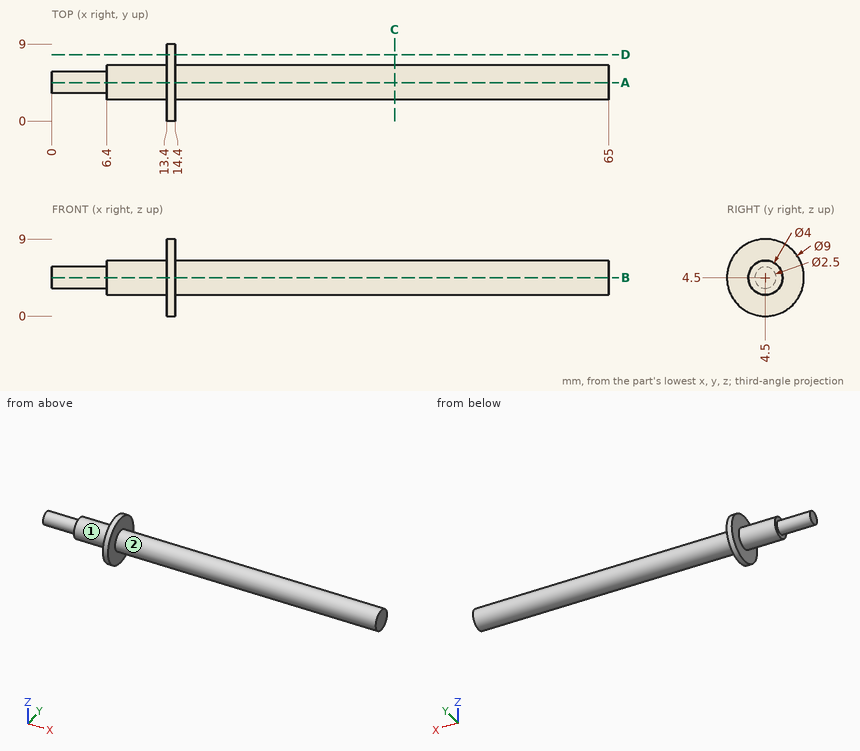
Geometry check sheet. Reference: drawing and pictorial views, mm from the part's lowest x, y, z. A direction names the side the tool comes from. Coordinates: 2 decimals unless noted, no trailing zeros. Write each loop counter-clockwise with the first axis right and the second up, starting at its lowest first coordinate (ties: lowest second). Pieces come first, ordered by that corner, then holes. Notation, with made-up numbers: (-2, 35.5) - (2, 35.5) arc R16 ccw to (2, 50.5) - close; hole circle Ø11 at (64, 48.5). An arc over 180 degrees is marked (long way). One line per question, with ' | ' between items. Start each with the question number.
1. Section check A-A (y = 4.5). Enter the section's corners in (x, z).
2. Material ranges on line 1 along X through (y, z) = (3, 6.5); line 2 along X through (y, z) = (5.75, 3.25); line 3 along Y through (x, z) = (49.5, 3.75), recorded low to high.
3. Gauge pin test, flat ends, axial feed: P1, Ø1.5, axis at y = 3.5, z = 5, coming from the -X side; P2, Ø1.5, axis at x = 20, y = 5.5, coming from the +Z side; P3, Ø1.5, axis at y = 6, z = 1.5, coming from the +X side; P4, Ø2, axis at x = 7.5, y = 4, coming from the -Z side. Record the tip position at first contact, or that the pin passes through.
4. Section check C-C (x = 40). Enter the section's corners in (y, z).
5. Access from +Z, -Z, +X, -X, +Y, -Y to the whole of each face (thin tool, end or side, straight path). Record for the marked faces 1 and 2.
6. Section check D-D (y = 7.75). Enter the section's corners in (x, z).
Computed values:
1) outline: (0, 3.25) - (6.4, 3.25) - (6.4, 2.5) - (13.4, 2.5) - (13.4, 0) - (14.4, 0) - (14.4, 2.5) - (65, 2.5) - (65, 6.5) - (14.4, 6.5) - (14.4, 9) - (13.4, 9) - (13.4, 6.5) - (6.4, 6.5) - (6.4, 5.75) - (0, 5.75) - close
2) line 1: 13.4 to 14.4 | line 2: 6.4 to 65 | line 3: 2.65 to 6.35
3) P1: x = 0 | P2: z = 6.48 | P3: x = 14.4 | P4: z = 2.5
4) outline: circle Ø4 at (4.5, 4.5)
5) face 1: -X | face 2: +X
6) outline: (13.4, 1.39) - (14.4, 1.39) - (14.4, 7.61) - (13.4, 7.61) - close
